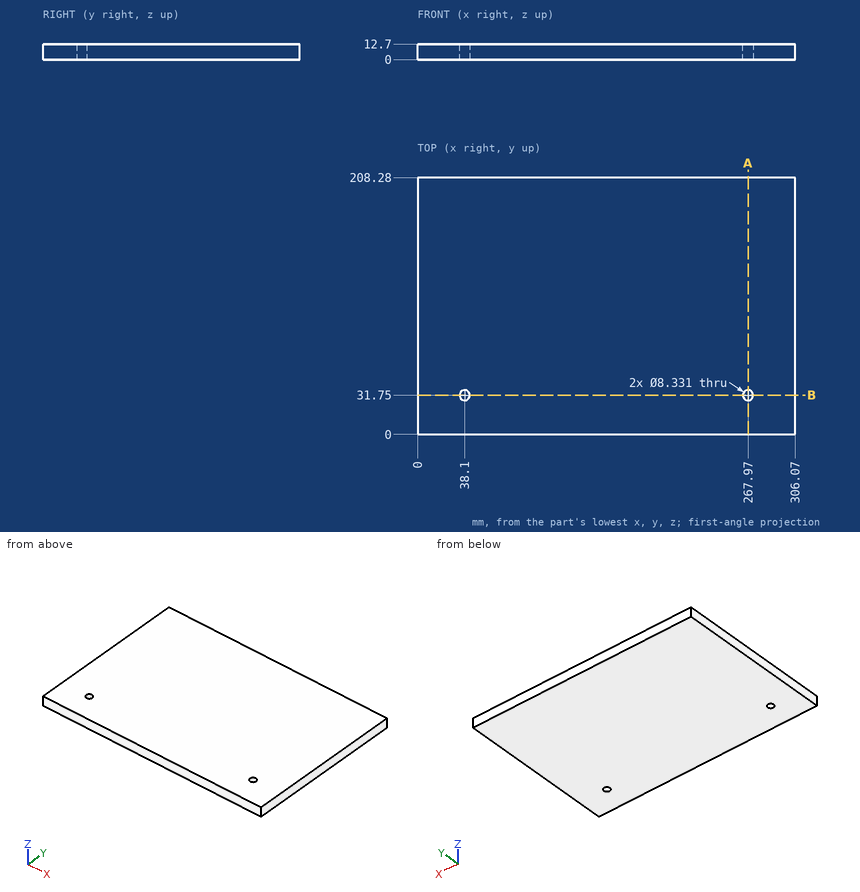
Drawing for the job (mm, zero at the part's lowest x, y, z). Give positions to 0.01 mm unless a question says otherwise; leave off trailing zeros. Order: outer loops, then holes, each group sorted by start corner. A loop starts at its lowest first (then second) coordinate and runs counter-clockwise, first axis right, second up. Notation, with made-up numbers: M 85,48 L 101,48 A26 ccw 101,66 Z; hole C 30.25,30.5 d5. An arc over 180 degrees is marked long. Put each result on its own line as item: value.
Item 1: Slice it at A-A, the plane x = 267.97. Write the cut outline in (y, z), plus the area to 3 significant figures.
From the geometry:
outline: M 0,0 L 27.58,0 L 27.58,12.7 L 0,12.7 Z; M 35.92,0 L 208.28,0 L 208.28,12.7 L 35.92,12.7 Z
area: 2,540 mm2
Item 2: Slice it at B-B, the plane y = 31.75. Write the cut outline in (x, z).
From the geometry:
outline: M 0,0 L 33.93,0 L 33.93,12.7 L 0,12.7 Z; M 42.27,0 L 263.8,0 L 263.8,12.7 L 42.27,12.7 Z; M 272.14,0 L 306.07,0 L 306.07,12.7 L 272.14,12.7 Z
Item 3: Probe line 1 (Y direction, x = 267.97, z = 7); line 2 (Y direction, x = 40.5, z = 8.25) (1 decimal). List the from-to ranges inside material, lowest first. Write a range as [from, to].
From the geometry:
line 1: y = [0, 27.58], [35.92, 208.28]
line 2: y = [0, 28.3], [35.2, 208.3]
